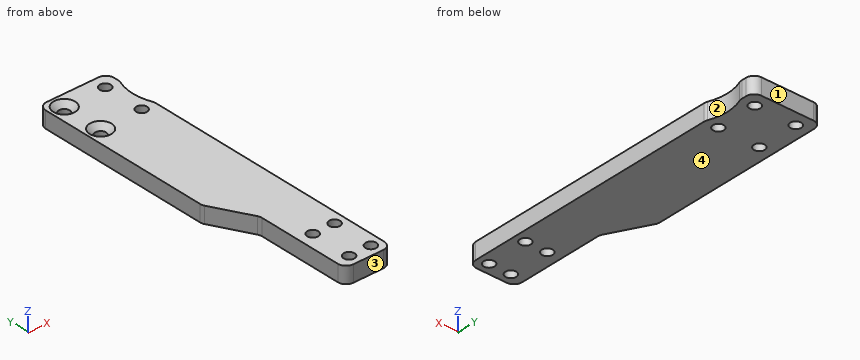
```python
from build123d import *

# Parameters (mm, degrees)
SKETCH_1_R          = 2
EXTRUDE_1_DEPTH     = 6
SKETCH_2_R          = 18
CUT_EXTRUDE_1_DEPTH = 6
SKETCH_3_W          = 2
SKETCH_3_H          = 20
SKETCH_3_W_2        = 23
SKETCH_3_H_2        = 10
CUT_EXTRUDE_2_DEPTH = 10
CUT_EXTRUDE_3_DEPTH = 10
EXTRUDE_2_DEPTH     = 6
SKETCH_6_W          = 15.770181782
SKETCH_6_H          = 14.407317349
EXTRUDE_3_DEPTH     = 6
SKETCH_7_R          = 2
CUT_EXTRUDE_4_DEPTH = 10
FILLET_1_R          = 3
SKETCH_8_R          = 2
CUT_EXTRUDE_5_DEPTH = 10
SKETCH_9_W          = 8
SKETCH_9_H          = 35
CUT_EXTRUDE_6_DEPTH = 10
CUT_EXTRUDE_7_DEPTH = 10
FILLET_2_R          = 3
CHAMFER_1_SIZE      = 2


with BuildPart() as part:
    # 草图1 → 凸台-拉伸1 (new body)
    with BuildSketch(Plane.XY):
        Polygon((12.5, 15), (18, 87.5), (18, 112.5), (-7, 112.5), (-7, 87.5), (-10.5, 15), (-12.5, 15), (-12.5, -15), (12.5, -15), align=None)
        with Locations((7.5, -6)):
            Circle(SKETCH_1_R, mode=Mode.SUBTRACT)
        with Locations((13, 92.5)):
            Circle(SKETCH_1_R, mode=Mode.SUBTRACT)
        with Locations((13, 107.5)):
            Circle(SKETCH_1_R, mode=Mode.SUBTRACT)
        with Locations((-2, 107.5)):
            Circle(SKETCH_1_R, mode=Mode.SUBTRACT)
        with Locations((7.5, 6)):
            Circle(SKETCH_1_R, mode=Mode.SUBTRACT)
        with Locations((-2, 92.5)):
            Circle(SKETCH_1_R, mode=Mode.SUBTRACT)
        with Locations((-0.5, 6)):
            Circle(SKETCH_1_R, mode=Mode.SUBTRACT)
        with Locations((-0.5, -6)):
            Circle(SKETCH_1_R, mode=Mode.SUBTRACT)
    extrude(amount=EXTRUDE_1_DEPTH)

    # 草图2 → 切除-拉伸1 (cut)
    with BuildSketch(Plane.XY.offset(6)):
        with Locations((34.5, 100)):
            Circle(SKETCH_2_R)
    extrude(amount=-CUT_EXTRUDE_1_DEPTH, mode=Mode.SUBTRACT)

    # 草图3 → 切除-拉伸2 (cut)
    with BuildSketch(Plane.XY.offset(6)):
        with Locations((-11.5, 5)):
            Rectangle(SKETCH_3_W, SKETCH_3_H)
        with Locations((1, -10)):
            Rectangle(SKETCH_3_W_2, SKETCH_3_H_2)
        with Locations((-11.5, -10)):
            Rectangle(SKETCH_3_W, SKETCH_3_H_2)
    extrude(amount=-CUT_EXTRUDE_2_DEPTH, mode=Mode.SUBTRACT)

    # 草图4 → 切除-拉伸3 (cut)
    with BuildSketch(Plane.XY.offset(6)):
        Polygon((-7, -5), (-7, 87.5), (-10.5, 15), (-10.5, -5), align=None)
    extrude(amount=-CUT_EXTRUDE_3_DEPTH, mode=Mode.SUBTRACT)

    # 草图5 → 凸台-拉伸2 (add)
    with BuildSketch(Plane.XY.offset(6)):
        Polygon((18, 87.5), (18, -5), (12.5, -5), (12.5, 15), align=None)
    extrude(amount=-EXTRUDE_2_DEPTH)

    # 草图6 → 凸台-拉伸3 (add)
    with BuildSketch(Plane.XY.offset(6)):
        with Locations((3.826559257, 2.203658675)):
            Rectangle(SKETCH_6_W, SKETCH_6_H)
    extrude(amount=-EXTRUDE_3_DEPTH)

    # 草图7 → 切除-拉伸4 (cut)
    with BuildSketch(Plane.XY.offset(6)):
        with Locations((6, -1)):
            Circle(SKETCH_7_R)
        with Locations((6, 14)):
            Circle(SKETCH_7_R)
        with Locations((-2, 14)):
            Circle(SKETCH_7_R)
        with Locations((-2, -1)):
            Circle(SKETCH_7_R)
    extrude(amount=-CUT_EXTRUDE_4_DEPTH, mode=Mode.SUBTRACT)

    # 圆角1
    fillet_1_edges = [part.edges().sort_by_distance(p)[0] for p in [
        (-7, -5, 3),
        (18, -5, 3),
        (-7, 112.5, 3),
        (18, 112.5, 3),
        (18, 107.193747285, 3),
        (18, 92.806252715, 3),
    ]]
    fillet(fillet_1_edges, radius=FILLET_1_R)

    # 草图8 → 切除-拉伸5 (cut)
    with BuildSketch(Plane.XY.offset(6)):
        with Locations((14, 14)):
            Circle(SKETCH_8_R)
        with Locations((14, -1)):
            Circle(SKETCH_8_R)
    extrude(amount=-CUT_EXTRUDE_5_DEPTH, mode=Mode.SUBTRACT)

    # 草图9 → 切除-拉伸6 (cut)
    with BuildSketch(Plane.XY.offset(6)):
        with Locations((-3, 12.5)):
            Rectangle(SKETCH_9_W, SKETCH_9_H)
    extrude(amount=-CUT_EXTRUDE_6_DEPTH, mode=Mode.SUBTRACT)

    # 草图10 → 切除-拉伸7 (cut)
    with BuildSketch(Plane.XY.offset(6)):
        Polygon((1, 30), (-7, 30), (-7, 45), align=None)
    extrude(amount=-CUT_EXTRUDE_7_DEPTH, mode=Mode.SUBTRACT)

    # 圆角2
    fillet_2_edges = [part.edges().sort_by_distance(p)[0] for p in [
        (1, 30, 3),
        (1, -5, 3),
        (-7, 45, 3),
    ]]
    fillet(fillet_2_edges, radius=FILLET_2_R)

    # 倒角1
    chamfer_1_edges = [part.edges().sort_by_distance(p)[0] for p in [
        (-4, 92.5, 6),
        (-4, 107.5, 6),
    ]]
    chamfer(chamfer_1_edges, length=CHAMFER_1_SIZE)


solid = part.part
```
Geometry check sheet. Reference: the model listing, model coordinates, mm. Face numbers are marked on the shaded views. Round coordinates to 2 decimals unless told otherwise and drop trailing zeros. Loops run counter-clockwise (first coordinate to the right, second up) from the corner with the lowest first, then second, coordinate; pieces in that order, holes last. Notation, with made-up numbers: M 1,-11.75 L 37,-11.75 A22 ccw 37,-4.75 Z; hole C -38,57 d4. An arc over 180 degrees is marked long. Return JSON: item names as keys, results as strings. Group by question number.
(1) Section check B-B, the plane x = -2. Enter the section's corners in (y, z) (3 decimals).
(2) Section check A-A, the plane y = 14. Enter the section's corners in (x, z), and give its area (3 significant figures).
(3) Go/stop test with flat-tipped pins: pin 1 (3.5 mm diameter, centred on x = 13, y = 107.5, fed in from -Z); pin 2 (3 mm diameter, centred on y = 28, z = 4, fed in from -X). Record where each tip stops, or that it passes through.
(4) Scan lines: line 1 along Y through (x, z) = (6, 3.8); line 2 along Y through (x, z) = (-2.75, 3.35); line 3 along X through (y, z) = (2, 2.1). Record each from-to range of solid material in increasing order. Write a range as [from, to].
(5) Section check C-C, the plane y = 101.5. Enter the section's corners in (x, z).
(6) Mould release check, pull along Y, two halves, no side actions. Record for the marked faces 1, 2, 3 and 4: pulls with the +Y half, pulls with the -Y half, needs draft (parallel to the pull), parting line crosses it, or undercut.
Data:
{
 "1": {"outline": "M 35.625,0 L 90.5,0 L 90.5,4 L 88.5,6 L 35.625,6 Z; M 94.5,0 L 105.5,0 L 105.5,4 L 103.5,6 L 96.5,6 L 94.5,4 Z; M 109.5,0 L 112.5,0 L 112.5,6 L 111.5,6 L 109.5,4 Z"},
 "2": {"outline": "M 1,0 L 4,0 L 4,6 L 1,6 Z; M 8,0 L 12,0 L 12,6 L 8,6 Z; M 16,0 L 18,0 L 18,6 L 16,6 Z", "area": "54.0 mm²"},
 "3": {"pin 1": "through", "pin 2": "x = 0.99"},
 "4": {"line 1": "[-5, -3], [1, 12], [16, 112.5]", "line 2": "[37.03, 90.65], [94.35, 105.65], [109.35, 112.5]", "line 3": "[1, 18]"},
 "5": {"outline": "M -7,0 L 16.56,0 L 16.56,6 L -7,6 Z"},
 "6": {"face 1": "pulls with the +Y half", "face 2": "undercut", "face 3": "pulls with the -Y half", "face 4": "needs draft"}
}
